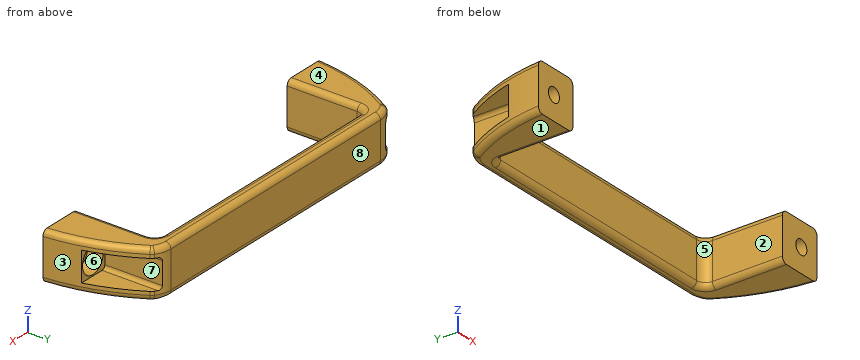
Autodesk Inventor part; units mm, degrees
ref_plane "YZ Plane" through (0, 0, 0) normal (1, 0, 0) x (0, 1, 0)
ref_plane "XZ Plane" through (0, 0, 0) normal (0, 1, 0) x (-1, 0, 0)
ref_plane "XY Plane" through (0, 0, 0) normal (0, 0, 1) x (1, 0, 0)
sketch "Sketch1" plane through (0, 0, 0) normal (0, 0, 1) x (1, 0, 0)
  line L0 (0.057, 44) -> (71, 44)
  line L1 (76.057, 52) -> (0.057, 52)
  line L2 (101.057, 0) -> (76, 0)
  line L3 (76, 0) -> (76, 39)
  arc A0 (101.057, 0) -> (85.6787, 47.8152) centre (-6.9827, -8.3672) ccw
  arc A1 (84.3966, 49.2278) -> (76.057, 52) centre (76.057, 38.0701) ccw
  arc A2 (85.6787, 47.8152) -> (84.3966, 49.2278) centre (81.4032, 45.2229) ccw
  line L4 (0.057, 44) -> (-71, 44)
  line L5 (-75.943, 52) -> (0.057, 52)
  line L6 (-100.943, 0) -> (-76, 0)
  line L7 (-76, 0) -> (-76, 39)
  arc A3 (-85.5646, 47.8152) -> (-100.943, 0) centre (7.0967, -8.3672) ccw
  arc A4 (-75.943, 52) -> (-84.2825, 49.2278) centre (-75.943, 38.0701) ccw
  arc A5 (-84.2825, 49.2278) -> (-85.5646, 47.8152) centre (-81.2891, 45.2229) ccw
  arc A6 (76, 39) -> (71, 44) centre (71, 39) ccw
  arc A7 (-71, 44) -> (-76, 39) centre (-71, 39) ccw
  line L8 (0, -20.5757) -> (0, 64.8833)
  point P0 (0, 0)
  point P1 (76, 44)
  point P2 (0.1141, 0)
  point P3 (-76, 44)
  dimension "d1" = 44
  dimension "d2" = 8
  dimension "d4" = 5
  dimension "d5" = 152
  dimension "d10" = 5
extrude "Extrusion1" add sketch "Sketch1" along normal mid plane 26.5
fillet "Fillet1" radius 3 14 edges at (-80.3371, 51.2888, 13.25) (-84.9915, 48.5832, 13.25) (-96.0624, 24.8109, 13.25) (80.4512, 51.2888, 13.25) (85.1056, 48.5832, 13.25) (96.1764, 24.8109, 13.25) (0.057, 52, 13.25) (80.4512, 51.2888, -13.25) (85.1056, 48.5832, -13.25) (96.1764, 24.8109, -13.25) (-80.3371, 51.2888, -13.25) (-84.9915, 48.5832, -13.25) (-96.0624, 24.8109, -13.25) (0.057, 52, -13.25)
fillet "Fillet2" radius 3 6 edges at (0, 44, 13.25) (76, 19.5, 13.25) (-76, 19.5, 13.25) (-76, 19.5, -13.25) (0, 44, -13.25) (76, 19.5, -13.25)
sketch "Sketch2" plane through (-75.943, 52, -10.25) normal (0, 1, 0) x (1, 0, 0)
  line L0 (-0.057, 0) -> (-0.057, -20.5)
  line L1 (151.943, 0) -> (151.943, -20.5)
  line L2 (177, 0) -> (177, -20.5)
  line L3 (177, -2) -> (158.943, -2)
  line L4 (156.943, -4) -> (156.943, -16.5)
  line L5 (158.943, -18.5) -> (177, -18.5)
  line L6 (177, -18.5) -> (177, -2)
  line L7 (159.0563, 3) -> (173.9908, 3)
  line L8 (173.9908, -23.5) -> (159.0563, -23.5)
  arc A0 (158.943, -2) -> (156.943, -4) centre (158.943, -4) ccw
  arc A1 (156.943, -16.5) -> (158.943, -18.5) centre (158.943, -16.5) ccw
  line L9 (-25, 0) -> (-25, -20.5)
  line L10 (-25, -2) -> (-7.057, -2)
  line L11 (-5.057, -4) -> (-5.057, -16.5)
  line L12 (-7.057, -18.5) -> (-25, -18.5)
  line L13 (-25, -18.5) -> (-25, -2)
  arc A2 (-5.057, -4) -> (-7.057, -2) centre (-7.057, -4) ccw
  arc A3 (-7.057, -18.5) -> (-5.057, -16.5) centre (-7.057, -16.5) ccw
  point P0 (75.943, -10.25)
  point P1 (166.5236, 3)
  dimension "d11" = 5
  dimension "d12" = 5
  dimension "d13" = 5
  dimension "d14" = 2
  dimension "d15" = 5
  dimension "d16" = 2
extrude "Extrusion2" cut sketch "Sketch2" against normal blind 33
sketch "Sketch3" plane through (-75.943, 19, -10.25) normal (0, 1, 0) x (1, 0, 0)
  line L0 (-65.4065, -10.25) -> (217.4065, -10.25)
  line L1 (-5.057, -4) -> (-5.057, -16.5)
  line L2 (75.943, 8.3065) -> (75.943, -28.8065)
  point P0 (75.943, -10.25)
  point P1 (-13.751, -10.25)
  dimension "d27" = 89.694
hole "Hole1" at (-89.694, 19, 0) direction (0, -1, 0) diameter 8 end through all counterbore diameter 15 counterbore depth 8.6
mirror "Mirror1" about plane through (0, 0, 0) normal (1, 0, 0) of "Hole1"
properties part number "Handle" material "Acetal Resin, Black"
Source: CAD feature listing. Evaluate the final solid. Frame: model axes, mm. Face numbers are marked on the shaded views. A direction names the side the tool comes from. Give positions to 0.01 mm unless a question says otherwise; leave off trailing zeros. Write item = value, one per line.
Q1. Material intervals for line 1 (X direction, y = 14.5, z = 5); line 2 (X direction, y = 2, z = 0); line 3 (X direction, y = 23, z = 5.5), sorted ascending. Write a range as from..to.
Data:
line_1 = -98.83..-95.28, -84.1..-76, 76..84.1, 95.28..98.94
line_2 = -100.77..-93.69, -85.69..-76, 76..85.69, 93.69..100.88
line_3 = -81..-76, 76..81
Q2. Pin query (flat end, axial travel): pin 1 (12 mm diameter, centred on x = -89.694, z = 0, fed in from +Y); pin 2 (10 mm diameter, centred on y = 38.5, z = -10, fed in from -X); pin 3 (6 mm diameter, centred on y = 11.5, z = 1.5, fed in from -X); pin 4 (10 mm diameter, centred on x = 79.5, z = 7.5, fed in from +Y). Return the tip coordinate at first contact, or that it passes through.
Data:
pin_1 = 10.4
pin_2 = -92.85
pin_3 = -99.95
pin_4 = 52
Q3. Pull-direction query (X, two-part tool) for the marked faces 1, 2 and 3; classes: released by +X, released by -X, zero draft, split by the parting line, or undercut.
Data:
face_1 = zero draft
face_2 = undercut
face_3 = released by +X
Q4. Cut plane A-A, the plane z = 0. State how many separate pieces and enclosed holes the cut face has, and give its area (3 significant figures).
Data:
separate_pieces = 3
enclosed_holes = 0
area = 2,030 mm^2
Q5. Set-up query: the marked faces 4, 5, 6, 7 and 8. Return all of +Z, -Z, +X, -X, +Y, -Y with unobstructed straight access to the full face (end or side cutting, diameter ignored); none if empty.
Data:
face_4 = +Z, +X, -X, +Y, -Y
face_5 = +Z, -Z, -Y
face_6 = +Y
face_7 = +X, +Y
face_8 = +Z, -Z, +X, -X, +Y
